Build history of the part. All positions in model axes, mm. A direction names the side the tool comes from. Coordinates: 2 decimals unless noted, no trailing zeros. Write each loop counter-clockwise with the first axis right and the second up, starting at its lowest first coordinate (ties: lowest second). Pieces come first, ordered by that corner, then holes. Notation, with made-up numbers: (53, 15) -> (112, 15) arc R32 cw to (112, 49) -> close; hole circle Ø9 at (-2.5, 71.25). An arc over 180 degrees is marked (long way). Write each question's results on one line, items separated by ' | '. Start each with the question number.
Q1. Saw through at B-B on y = 50. Give the cut face in (x, z).
Q2. Saw through at D-D on x = 89.5. Give the cut face in (y, z).
Q3. Two-plate mould, pull along Y, no slides. Class faces 4 (the face through (115, 46.99, 38)), 5 (the face through (41.4, 23.22, 37.57)), 6 (the face through (83.82, 61, 50)): released by +Y, released by -Y, zero draft, split by the parting line, or undercut.
Q4. Drill centre lines: line 1 (Y direction, x = 38.1, z = 40); line 2 (X direction, y = 38, z = 19); line 3 (Z direction, x = 151.5, y = 22.5). Where is each one in solid material? Low to high.
Q5. Saw through at A-A on z = 21. Give the cut face in (x, y).
Q6. Drop flat-ended pins along their axis: pin 1 Ø6 at (x, y) = (35, 51) entering from +Z; pin 2 Ø9 at (x, y) = (114, 17.5) entering from +Z; pin 3 Ø9 at (y, z) = (63.5, 40.5) entering from +X; pin 4 Ø6 at (y, z) = (10, 31.5) entering from -X. Give the stop position or say it passes through.
Q7. Saw through at C-C on z = 47.5. Give the cut face in (x, y).
Q8. Tool access for faces 1 (the face through (140, 62, 22.86)), 2 (the face through (83.82, 14, 50)), 3 (the face through (198.12, 38, 11)): list every direction of +Z, -Z, +X, -X, +Y, -Y with a clear straight run to the whole face (end or side of a thin tool).
from build123d import *

# Parameters (mm, degrees)
F1_DEPTH = 76.2
F3_D     = 30.48
F2_W     = 114.3
F2_H     = 29.21
F4_DEPTH = 53.34
F6_DEPTH = 17.78
F8_DEPTH = 22.86


with BuildPart() as f1:
    # F0 (on Top) → F1 (new body)
    with BuildSketch(Plane.XY):
        with BuildLine():
            ThreePointArc((0, 38.1), (11.159232, 11.159232), (38.1, 0))
            Line((38.1, 0), (198.12, 0))
            Line((198.12, 0), (198.12, 76.2))
            Line((198.12, 76.2), (38.1, 76.2))
            ThreePointArc((38.1, 76.2), (11.159232, 65.040768), (0, 38.1))
        make_face()
    extrude(amount=F1_DEPTH)

    # F3 (through all)
    with Locations(Plane.XY.offset(76.2)):
        with Locations((38.1, 38.1)):
            Hole(F3_D / 2)

    # F2 (on face) → F4 (cut)
    with BuildSketch(Plane.XY.offset(76.2)):
        with Locations((140.97, 61.595)):
            Rectangle(F2_W, F2_H)
        with Locations((140.97, 14.605)):
            Rectangle(F2_W, F2_H)
    extrude(amount=-F4_DEPTH, mode=Mode.SUBTRACT)

    # F5 (on face) → F6 (cut)
    with BuildSketch(Plane.XZ.offset(-29.21)):
        Polygon((198.12, 76.2), (83.82, 76.2), (198.12, 22.86), align=None)
    extrude(amount=-F6_DEPTH, mode=Mode.SUBTRACT)

    # F7 (on face) → F8 (cut)
    with BuildSketch(Plane(origin=(0, 0, 0), x_dir=(1, 0, 0), z_dir=(0, 0, -1))):
        Polygon((198.12, 0), (175.26, 0), (198.12, -22.86), align=None)
        Polygon((198.12, -76.2), (198.12, -53.34), (175.26, -76.2), align=None)
    extrude(amount=-F8_DEPTH, mode=Mode.SUBTRACT)


solid = f1.part
Returned:
1) outline: (1.91, 0) -> (28.58, 0) -> (28.58, 76.2) -> (1.91, 76.2) -> close; (47.62, 0) -> (198.12, 0) -> (198.12, 22.86) -> (83.82, 22.86) -> (83.82, 76.2) -> (47.62, 76.2) -> close
2) outline: (0, 0) -> (76.2, 0) -> (76.2, 22.86) -> (46.99, 22.86) -> (46.99, 73.55) -> (29.21, 73.55) -> (29.21, 22.86) -> (0, 22.86) -> close
3) face 4: released by +Y | face 5: undercut | face 6: zero draft
4) line 1: y = 0 to 22.86, 53.34 to 76.2 | line 2: x = 0 to 22.86, 53.34 to 198.12 | line 3: z = 0 to 22.86
5) outline: (0, 38.1) arc R38.1 ccw to (38.1, 0) -> (175.26, 0) -> (198.12, 22.86) -> (198.12, 53.34) -> (175.26, 76.2) -> (38.1, 76.2) arc R38.1 ccw to start; hole circle Ø30.48 at (38.1, 38.1)
6) pin 1: stops at z = 76.2 | pin 2: stops at z = 22.86 | pin 3: stops at x = 83.82 | pin 4: stops at x = 9.44
7) outline: (0, 38.1) arc R38.1 ccw to (38.1, 0) -> (83.82, 0) -> (83.82, 29.21) -> (145.32, 29.21) -> (145.32, 46.99) -> (83.82, 46.99) -> (83.82, 76.2) -> (38.1, 76.2) arc R38.1 ccw to start; hole circle Ø30.48 at (38.1, 38.1)
8) face 1: +Z, +X, +Y | face 2: +Z, +X, -Y | face 3: +Z, -Z, +X, +Y, -Y
